Source: CAD feature listing. Evaluate the final solid. Frame: model axes, mm. A direction names the side the tool comes from. Give positions to 0.01 mm unless a question says otherwise; leave off trailing zeros. Loops run counter-clockwise (first coordinate to the right, second up) from the corner with the lowest first, then second, coordinate; pieces in that order, holes last. Notation, with made-up numbers: (-2, -33.75) -> (22, -33.75) arc R25 ccw to (22, -16.75) -> close; hole circle Ø4 at (18, 65). An arc over 180 degrees is marked (long way). Return JSON: item names as keys, results as strings. Group by question number.
(1) Access query for faces 1 (the face through (1, -0.452, 3)), 2 (the face through (6.39, 8.11, 5.01)), 3 (the face through (6, 9.548, 5)). Directions: +Z, -Z, +X, -X, +Y, -Y. A direction counts if a zero-diameter tool reaches every point of the face in a straight line with its end or side. Return the directions, or none.
(2) Cut plane B-B on z = 5.08. Return loops of the section in (x, y), then the cut area to 3 significant figures.
(3) Draft query along Z for faces 4 (the face through (-1.336, -3.753, 2.662)), 5 (the face through (3, 1, 10.16)), 6 (the face through (-6.26, 1, 5)). Return one class per face: released by +Z, released by -Z, zero draft, split by the parting line, or undercut.
(4) Pin query (flat end, axial travel): pin 1 (3.5 mm diameter, centred on x = 13.68, z = 5.08, fed in from -Y); pin 2 (6 mm diameter, centred on x = -2, z = 3, fed in from +Y); pin 3 (3 mm diameter, centred on x = 12.5, z = 5.5, fed in from +Y). Return the tip coordinate at first contact, or that it passes through.
(5) Cut plane A-A on y = -1. Return loops of the section in (x, z), then the cut area to 3 significant figures.
(6) Cut plane C-C on x = 11.75. Return loops of the section in (y, z), then the cut area to 3 significant figures.
(7) Cut plane D-D on z = 9. Return loops of the section in (x, y).
(8) Ray query, line 1 (Z direction, x = 13.5, y = 2); line 2 (X direction, y = -3.5, z = 5.08); line 3 (X direction, y = -3, z = 2.25). Return the intervals inside material, ascending. Write a range as from..to.
Autodesk Inventor part; units mm, degrees
ref_plane "YZ Plane" through (0, 0, 0) normal (1, 0, 0) x (0, 1, 0)
ref_plane "XZ Plane" through (0, 0, 0) normal (0, 1, 0) x (-1, 0, 0)
ref_plane "XY Plane" through (0, 0, 0) normal (0, 0, 1) x (1, 0, 0)
sketch "Sketch1" plane through (0, 0, 0) normal (0, 0, 1) x (1, 0, 0)
  line L0 (-6.2599, 9.5475) -> (19.1401, 9.5475)
  line L1 (19.1401, 9.5475) -> (19.1401, -6.9625)
  line L2 (19.1401, -6.9625) -> (-6.2599, -6.9625)
  line L3 (-6.2599, -6.9625) -> (-6.2599, 9.5475)
  point P0 (0, 0)
  dimension "d0" = 25.4
  dimension "d1" = 16.51
extrude "Plate1" add sketch "Sketch1" along normal blind 10.16
sketch "Sketch4" plane through (-6.2599, -6.9625, 0) normal (0, -1, 0) x (1, 0, 0)
  circle A0 centre (5.461, 5.08) radius 2.4765
  circle A1 centre (19.939, 5.08) radius 2.4765
  line L0 (25.4, 0) -> (25.4, 10.16)
  line L1 (0, 0) -> (0, 10.16)
  line L2 (25.4, 10.16) -> (0, 10.16)
  circle A2 centre (5.461, 5.08) radius 2.4765
  circle A3 centre (19.939, 5.08) radius 2.4765
  dimension "d30" = 4.953
  dimension "d37" = 5.461
  dimension "d38" = 5.461
extrude "Extrusion1" cut sketch "Sketch4" against normal blind 14
sketch "Sketch5" plane through (-6.2599, 9.5475, 0) normal (0, 1, 0) x (1, 0, 0)
  circle A0 centre (5.461, -5.08) radius 2.4765
  circle A1 centre (5.461, -5.08) radius 2.9464
  circle A2 centre (19.939, -5.08) radius 2.4765
  circle A3 centre (19.939, -5.08) radius 2.9464
  line L0 (25.4, 0) -> (25.4, -10.16)
  line L1 (0, 0) -> (0, -10.16)
  point P0 (6.2599, 0)
extrude "Extrusion2" cut sketch "Sketch5" against normal blind 10
sketch "Sketch6" plane through (0, 0, 0) normal (0, 0, -1) x (-1, 0, 0)
  line L0 (-19.1401, 9.5475) -> (-19.1401, -6.9625)
  line L1 (6.2599, 9.5475) -> (-19.1401, 9.5475)
  line L2 (6.2599, -6.9625) -> (6.2599, 9.5475)
  line L3 (6.2599, 1.2925) -> (-19.1401, 1.2925) construction
  line L4 (-6.4401, 6.0296) -> (-6.4401, -3.4446) construction
  line L5 (-19.1401, -6.9625) -> (6.2599, -6.9625)
  line L6 (-8.5229, 6.0296) -> (-8.5229, -3.4446)
  line L7 (-4.3573, -3.4446) -> (-4.3573, 6.0296)
  arc A0 (-4.3573, 6.0296) -> (-8.5229, 6.0296) centre (-6.4401, 6.0296) ccw
  arc A1 (-8.5229, -3.4446) -> (-4.3573, -3.4446) centre (-6.4401, -3.4446) ccw
  point P0 (-6.4401, 1.2925)
  dimension "d26" = 13.6398
  dimension "d27" = 2.0828
extrude "Extrusion3" cut sketch "Sketch6" against normal through all contours A0 L7 A1 L6
sketch "Sketch7" plane through (-6.2599, 9.5475, 0) normal (0, 1, 0) x (1, 0, 0)
  circle A0 centre (5.461, -5.08) radius 2.9464
  circle A1 centre (5.461, -5.08) radius 2.4765
  circle A2 centre (19.939, -5.08) radius 2.4765
  circle A3 centre (19.939, -5.08) radius 2.4765
  point P0 (6.2599, 0)
extrude "Extrusion4" cut sketch "Sketch7" against normal up to next contours A1 | A2
sketch "Sketch8" plane through (0, 0, 0) normal (0, 0, -1) x (-1, 0, 0)
  arc A0 (-8.5229, -3.4446) -> (-4.3573, -3.4446) centre (-6.4401, -3.4446) ccw
  line L0 (-8.5229, -3.4446) -> (-8.5229, 6.0296)
  line L1 (-6.4401, 1.2925) -> (-3.3921, 1.2925) construction
  line L2 (-6.4401, 1.2925) -> (-9.4881, 1.2925) construction
  line L3 (-3.3921, 1.2925) -> (-3.3921, 9.5475) construction
  line L4 (6.2599, 9.5475) -> (-19.1401, 9.5475)
  point P0 (0, 0)
  dimension "d41" = 3.048
  dimension "d42" = 3.048
equation "\"BendRadius\" = Thickness"
equation "\"BendReliefWidth\" = Thickness"
equation "\"BendReliefDepth\" = 0.5 * Thickness"
equation "\"CornerReliefSize\" = 4 * Thickness"
equation "\"MinimumRemnant\" = 2 * Thickness"
equation "\"TransitionRadius\" = BendRadius"
equation "\"JacobiRadiusSize\" = Thickness"
equation "\"GapSize\" = Thickness"
equation "\"d2\" = BendRadius"
properties part number "Hew Sensor Mount 2017"
Answers:
{
 "1": {"face 1": "+Y", "face 2": "+Z, -Z", "face 3": "+Z, -Z, +X, -X, +Y"},
 "2": {"outline": "(-6.26, -6.96) -> (-3.28, -6.96) -> (-3.28, -0.45) -> (-3.75, -0.45) -> (-3.75, 9.55) -> (-6.26, 9.55) -> close; (1.68, -6.96) -> (11.2, -6.96) -> (11.2, -0.45) -> (10.73, -0.45) -> (10.73, 9.55) -> (2.15, 9.55) -> (2.15, -0.45) -> (1.68, -0.45) -> close; (16.16, -6.96) -> (19.14, -6.96) -> (19.14, 9.55) -> (16.63, 9.55) -> (16.63, -0.45) -> (16.16, -0.45) -> close; hole (4.36, -3.44) arc R2.08 ccw to (8.52, -3.44) -> (8.52, 6.03) arc R2.08 ccw to (4.36, 6.03) -> close", "area": "184 mm²"},
 "3": {"face 4": "undercut", "face 5": "released by +Z", "face 6": "zero draft"},
 "4": {"pin 1": "through", "pin 2": "y = 9.55", "pin 3": "y = -0.45"},
 "5": {"outline": "(-6.26, 0) -> (4.36, 0) -> (4.36, 10.16) -> (-6.26, 10.16) -> close; (8.52, 0) -> (19.14, 0) -> (19.14, 10.16) -> (8.52, 10.16) -> close; hole circle Ø4.95 at (-0.8, 5.08); hole circle Ø4.95 at (13.68, 5.08)", "area": "177 mm²"},
 "6": {"outline": "(-6.96, 0) -> (9.55, 0) -> (9.55, 2.85) -> (-0.45, 2.85) -> (-0.45, 3.53) -> (-6.96, 3.53) -> close; (-6.96, 6.63) -> (-0.45, 6.63) -> (-0.45, 7.31) -> (9.55, 7.31) -> (9.55, 10.16) -> (-6.96, 10.16) -> close", "area": "103 mm²"},
 "7": {"outline": "(-6.26, -6.96) -> (19.14, -6.96) -> (19.14, 9.55) -> (-6.26, 9.55) -> close; hole (4.36, -3.44) arc R2.08 ccw to (8.52, -3.44) -> (8.52, 6.03) arc R2.08 ccw to (4.36, 6.03) -> close"},
 "8": {"line 1": "0..2.14, 8.02..10.16", "line 2": "-6.26..-3.28, 1.68..4.36, 8.52..11.2, 16.16..19.14", "line 3": "-6.26..4.36, 8.52..19.14"}
}
